from build123d import *

# Parameters (mm, degrees)
F1_DEPTH  = 9.5
F2_W      = 9.5
F2_H      = 119.5
F2_H_2    = 9.5
F2_W_2    = 93
F3_DEPTH  = 48
F5_DEPTH  = 9.5
F6_R      = 2.5
F7_DEPTH  = 25.4
F8_W      = 15
F8_H      = 12.7057269514
F9_DEPTH  = 9.501
F10_W     = 260.0785551071
F10_H     = 9.5
F11_DEPTH = 48
F12_SIZE  = 2


# Not quite as in the source:
# - a feature names something its author has since deleted; it is built from what else it names


with BuildPart() as f1:
    # F0 (on Top) → F1 (new body)
    with BuildSketch(Plane.XY):
        Polygon((0, 129), (0, 0), (556, 0), (556, 43), (438, 43), (438, 114.0399202704), (426, 114.0399202704), (426, 33.5), (310, 33.5), (310, 83.1064879894), (302.5, 83.1064879894), (302.5, 129), align=None)
    extrude(amount=F1_DEPTH)

    # F2 (on face) → F3 (join)
    with BuildSketch(Plane.XY.offset(9.5)):
        with Locations((4.75, 69.25)):
            Rectangle(F2_W, F2_H)
        with Locations((4.75, 4.75)):
            Rectangle(F2_W, F2_H_2)
        with Locations((56, 4.75)):
            Rectangle(F2_W_2, F2_H_2)
        with Locations((107.25, 69.25)):
            Rectangle(F2_W, F2_H)
        with Locations((107.25, 4.75)):
            Rectangle(F2_W, F2_H_2)
    extrude(amount=F3_DEPTH)

    # F4 (on face) → F5 (join)
    with BuildSketch(Plane.XY.offset(9.5)):
        Polygon((426, 129), (302.5, 129), (302.5, 83.1064879894), (310, 83.1064879894), (310, 33.5), (426, 33.5), align=None)
    extrude(amount=-F5_DEPTH)

    # F6 (on face) → F7 (cut)
    with BuildSketch(Plane.XY.offset(9.5)):
        with BuildLine():
            ThreePointArc((244.5, 64.5), (242, 67), (239.5, 64.5))
            Line((239.5, 64.5), (244.5, 64.5))
        make_face()
        with BuildLine():
            Line((244.5, 64.5), (239.5, 64.5))
            ThreePointArc((239.5, 64.5), (242, 62), (244.5, 64.5))
        make_face()
        with Locations((376, 64.5)):
            Circle(F6_R)
    extrude(amount=-F7_DEPTH, mode=Mode.SUBTRACT)

    # F8 (on face) → F9 (cut, through all)
    with BuildSketch(Plane.XY.offset(9.5)):
        with Locations((463.5, 36.6471365243)):
            Rectangle(F8_W, F8_H)
        with Locations((528.5, 36.6471365243)):
            Rectangle(F8_W, F8_H)
    extrude(amount=-F9_DEPTH, mode=Mode.SUBTRACT)

    # F10 (on face) → F11 (join)
    with BuildSketch(Plane.XY.offset(9.5)):
        with Locations((425.9607224464, 4.75)):
            Rectangle(F10_W, F10_H)
    extrude(amount=F11_DEPTH)

    # F12
    f12_edges = [f1.edges().sort_by_distance(p)[0] for p in [
        (0, 64.5, 57.5),
        (9.5, 69.25, 57.5),
        (56, 0, 57.5),
        (56, 9.5, 57.5),
        (102.5, 69.25, 57.5),
        (112, 64.5, 57.5),
        (107.25, 129, 57.5),
        (4.75, 129, 57.5),
        (56, 129, 9.5),
        (269, 129, 9.5),
        (203.960722, 0, 9.5),
        (425.960722, 0, 57.5),
        (425.960722, 9.5, 57.5),
        (556, 4.75, 57.5),
        (438, 78.51996, 9.5),
        (426, 121.51996, 9.5),
        (432, 114.03992, 9.5),
        (112, 0, 33.5),
        (0, 0, 28.75),
        (295.921445, 4.75, 57.5),
        (295.921445, 0, 33.5),
        (556, 0, 28.75),
    ]]
    chamfer(f12_edges, length=F12_SIZE)


solid = f1.part
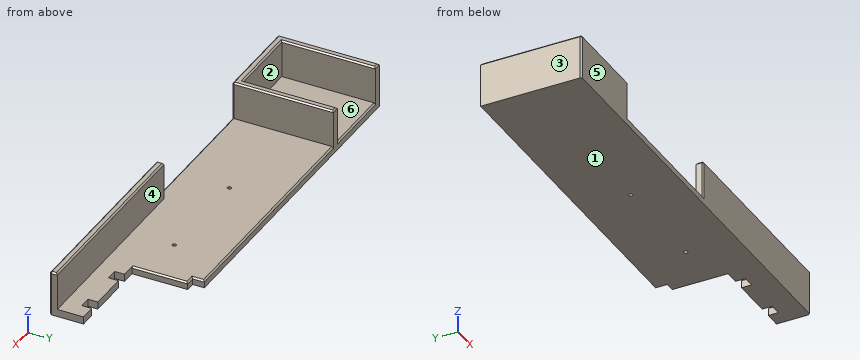
Here's how the part is built. I have some questions about the finished solid (model axes, mm). Face numbers are marked on the shaded views. A direction names the side the tool comes from. Coordinates: 2 decimals unless noted, no trailing zeros. Write each loop counter-clockwise with the first axis right and the second up, starting at its lowest first coordinate (ties: lowest second). Pieces come first, ordered by that corner, then holes.
Item 1: I want a section at B-B on x = 404.5. Write out the boundary of the cut face in (y, z), and give its area (3 significant figures).
Item 2: I want a section at C-C on y = 19. Write out the boundary of the cut face in (x, z), and give its area (3 significant figures).
Item 3: On a 3-axis mill with a long thin cutter (end or side, diameter ignored), from which of +Z, -Z, +X, -X, +Y, -Y can I reach the whole of each face in a straight line? I mean the marked faces 4, 5 and 6. Say none if no direction works.
Item 4: If we mould it in two halves opening along X, with no side actions, what happens to the marked faces 1, 2 and 3? For each: +X half, -X half, draft (parallel to the pull), parting line (faces both ways), or undercut.
Item 5: Will these pins go through, and if not, where does the flat tip stop? pin 1 (4 mm diameter, centred on y = 55.5, z = 29, fed in from +X); pin 2 (7.5 mm diameter, centred on x = 446.5, z = 4.5, fed in from +Y); pin 3 (8 mm diameter, centred on x = 432.5, z = 4.5, fed in from +Y); pin 4 (1 mm diameter, centred on x = 114, z = 13, fed in from +Y).
Item 6: I want a section at D-D on y = 104. Write out the boundary of the cut face in (x, z).
Item 7: I want a section at A-A on z = 14.5. Write out the boundary of the cut face in (x, y).
Item 8: If I drill on line 1 (X direction, y = 64, z = 3); line 2 (X direction, y = 107, z = 43); line 3 (Y direction, x = 376, z = 6), over which ranges is the centre line in solid material (lowest first)?
Findings below:
1. outline: (0, 0) - (129, 0) - (129, 7.5) - (127, 9.5) - (9.5, 9.5) - (9.5, 55.5) - (7.5, 57.5) - (2, 57.5) - (0, 55.5) - close
1. area: 1,680 mm2
2. outline: (0, 0) - (556, 0) - (556, 9.5) - (112, 9.5) - (112, 55.5) - (110, 57.5) - (104.5, 57.5) - (102.5, 55.5) - (102.5, 9.5) - (9.5, 9.5) - (9.5, 55.5) - (7.5, 57.5) - (2, 57.5) - (0, 55.5) - close
2. area: 6,190 mm2
3. face 4: +Z, +X, +Y
3. face 5: +Z, -Z, +X, -X, -Y
3. face 6: +Z, +Y
4. face 1: draft
4. face 2: undercut
4. face 3: -X half
5. pin 1: stops at x = 112
5. pin 2: stops at y = 43
5. pin 3: stops at y = 114.04
5. pin 4: passes through
6. outline: (0, 0) - (438, 0) - (438, 7.5) - (436, 9.5) - (112, 9.5) - (112, 55.5) - (110, 57.5) - (104.5, 57.5) - (102.5, 55.5) - (102.5, 9.5) - (9.5, 9.5) - (9.5, 55.5) - (7.5, 57.5) - (2, 57.5) - (0, 55.5) - close
7. outline: (0, 2) - (2, 0) - (110, 0) - (112, 2) - (112, 129) - (102.5, 129) - (102.5, 9.5) - (9.5, 9.5) - (9.5, 129) - (0, 129) - close; (295.92, 2) - (297.92, 0) - (554, 0) - (556, 2) - (556, 9.5) - (295.92, 9.5) - close
8. line 1: x = 0 to 239.55, 244.45 to 373.55, 378.45 to 438
8. line 2: x = 0 to 9.5, 102.5 to 112
8. line 3: y = 0 to 62, 67 to 129
